Part model, mm, in its own coordinate system. Face numbers are marked on the shaded views. Give positions to 0.01 mm unless a question says otherwise; leave off trailing zeros. Order: outer loops, then holes, each group sorted by start corner. A loop starts at its lowest first (then second) coordinate and runs counter-clockwise, first axis right, second up. Notation, with made-up numbers: (41.5, 60.25) -> (59.5, 60.25) arc R18 cw to (59.5, 85.25) -> close; hole circle Ø3 at (-19, 64.25). An arc over 180 degrees is marked (long way). Write item = value, one per line. Start each with the question number.
(1) Probe line 1 along X through (y, z) = (0, 48); line 2 along Y through (x, z) = (0, 44); line 3 along Z through (x, y) = (-20.5, -15). List the from-to ranges inside material, lowest first. Write a range as from..to.
(2) Saw through at B-B, the plane x = 0. List the corners of the cut face in (y, z), then the cut area to 3 significant figures.
(3) Saw through at A-A, the plane y = 0. List the corners of the cut face in (x, z).
(4) Two-plate mould, pull along Y, no slides. Class the marked faces 1, 2, 3 and 4: pulls with the +Y half, pulls with the -Y half, needs draft (parallel to the pull), parting line crosses it, or undercut.
(5) Saw through at C-C, the plane z = 63. List the corners of the cut face in (x, y).
(6) Flat gauge pins, fed straight in: pin 1 (5 mm diameter, centred on x = -43, y = -26, fed in from +Z); pin 2 (21 mm diameter, centred on x = 6, z = 69.5, fed in from -Y); pin 3 (3 mm diameter, centred on y = 15.5, z = 77, fed in from -X). Where does each tip first touch, or does it go through?
from build123d import *

# Parameters (mm, degrees)
F1_DEPTH = 20
F3_DEPTH = 70


with BuildPart() as f1:
    # F0 (on Top) → F1 (new body)
    with BuildSketch(Plane.XY):
        with BuildLine():
            Line((40, 44.72136), (-40, 44.72136))
            ThreePointArc((-40, 44.72136), (0, -60), (40, 44.72136))
        make_face()
    extrude(amount=F1_DEPTH)

    # F2 (on face) → F3 (join)
    with BuildSketch(Plane.XY.offset(20)):
        with BuildLine():
            Line((40, 44.72136), (-40, 44.72136))
            ThreePointArc((-40, 44.72136), (0, -60), (40, 44.72136))
        make_face()
        with BuildLine():
            ThreePointArc((38.837201, 41.72136), (0, -57), (-38.837201, 41.72136))
            Line((-38.837201, 41.72136), (38.837201, 41.72136))
        make_face(mode=Mode.SUBTRACT)
    extrude(amount=F3_DEPTH)


solid = f1.part
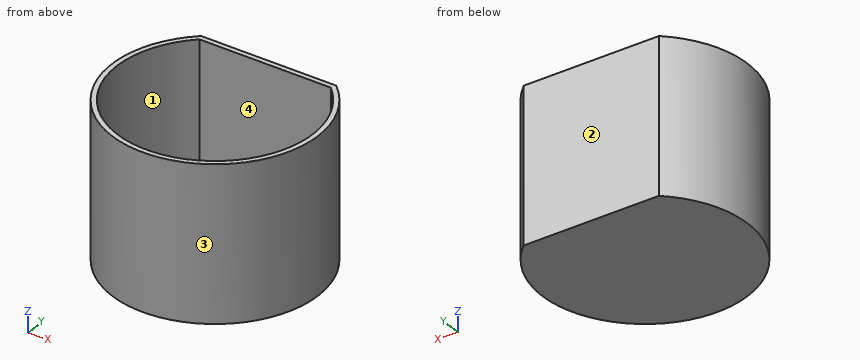
Results list:
q1.line_1 = -60..-57, 57..60
q1.line_2 = -60..-57, 41.72..44.72
q1.line_3 = 0..20
q2.outline = (-60, 0) -> (44.72, 0) -> (44.72, 90) -> (41.72, 90) -> (41.72, 20) -> (-57, 20) -> (-57, 90) -> (-60, 90) -> close
q2.area = 2,510 mm^2
q3.outline = (-60, 0) -> (60, 0) -> (60, 90) -> (57, 90) -> (57, 20) -> (-57, 20) -> (-57, 90) -> (-60, 90) -> close
q4.face_1 = undercut
q4.face_2 = pulls with the +Y half
q4.face_3 = parting line crosses it
q4.face_4 = undercut
q5.outline = (-40, 44.72) arc R60 ccw (long way) to (40, 44.72) -> close; hole (-38.84, 41.72) arc R57 ccw (long way) to (38.84, 41.72) -> close
q6.pin_1 = 20
q6.pin_2 = -60
q6.pin_3 = -58.34
